For this review, take the finished solid that the model builds, in its own axes (mm). Coordinates: 2 decimals unless noted, no trailing zeros. Write each loop counter-clockwise with the first axis right and the second up, starting at its lowest first coordinate (ties: lowest second). Pieces come first, ordered by that corner, then holes.
```python
from build123d import *

# Parameters (mm, degrees)
PAD_DEPTH     = 3
SKETCH002_R   = 1.95
HOLE_DEPTH    = 3.001
SKETCH_R      = 15
HOLE001_DEPTH = 3.001
SKETCH003_R   = 1.95
HOLE002_DEPTH = 3.001
SKETCH004_R   = 5.7
SKETCH004_R_2 = 4.8
POCKET_DEPTH  = 3.001


with BuildPart() as part:
    # Sketch001 → Pad (new body)
    with BuildSketch(Plane.XY):
        with BuildLine():
            Line((11.5, 190), (11.5, 20))
            ThreePointArc((11.5, 20), (12.525126, 17.525126), (15, 16.5))
            Line((15, 16.5), (120, 16.5))
            ThreePointArc((120, 16.5), (122.474874, 17.525126), (123.5, 20))
            Line((123.5, 20), (123.5, 190))
            ThreePointArc((123.5, 190), (122.474874, 192.474874), (120, 193.5))
            Line((120, 193.5), (15, 193.5))
            ThreePointArc((15, 193.5), (12.525126, 192.474874), (11.5, 190))
        make_face()
    extrude(amount=PAD_DEPTH)

    # Sketch002 → Hole (cut, through all)
    with BuildSketch(Plane.XY):
        with Locations((50, 87.5)):
            Circle(SKETCH002_R)
        with Locations((85, 87.5)):
            Circle(SKETCH002_R)
        with Locations((85, 122.5)):
            Circle(SKETCH002_R)
        with Locations((50, 122.5)):
            Circle(SKETCH002_R)
    extrude(amount=HOLE_DEPTH, mode=Mode.SUBTRACT)

    # Sketch → Hole001 (cut, through all)
    with BuildSketch(Plane.XY):
        with Locations((67.5, 105)):
            Circle(SKETCH_R)
    extrude(amount=HOLE001_DEPTH, mode=Mode.SUBTRACT)

    # Sketch003 → Hole002 (cut, through all)
    with BuildSketch(Plane.XY):
        with Locations((90, 83)):
            Circle(SKETCH003_R)
        with Locations((45, 83)):
            Circle(SKETCH003_R)
        with Locations((45, 128)):
            Circle(SKETCH003_R)
        with Locations((90, 128)):
            Circle(SKETCH003_R)
    extrude(amount=HOLE002_DEPTH, mode=Mode.SUBTRACT)

    # Sketch004 → Pocket (cut, through all)
    with BuildSketch(Plane.XY):
        with Locations((45, 35)):
            Circle(SKETCH004_R)
        with Locations((65, 35)):
            Circle(SKETCH004_R_2)
    extrude(amount=POCKET_DEPTH, mode=Mode.SUBTRACT)


solid = part.part
```
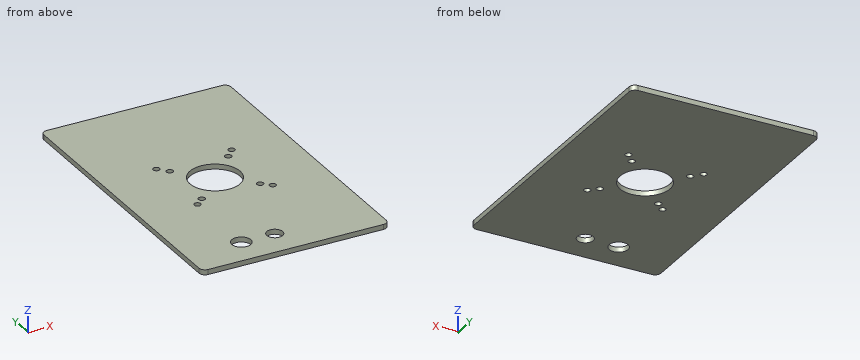
Q1. For probe 1 along Y at (x, z) = (45, 1.6); probe 2 along Y at (x, z) = (85, 1.2); probe 3 along Y at (x, z) = (90, 1.7), list the stretches that pass through material, from the lowest coordinate up.
Ans:
probe 1: y = 16.5 to 29.3, 40.7 to 81.05, 84.95 to 126.05, 129.95 to 193.5
probe 2: y = 16.5 to 85.55, 89.45 to 120.55, 124.45 to 193.5
probe 3: y = 16.5 to 81.05, 84.95 to 126.05, 129.95 to 193.5
Q2. Add section C-C (y = 83). State the section outline as (x, z) points.
Ans:
outline: (11.5, 0) - (43.05, 0) - (43.05, 3) - (11.5, 3) - close; (46.95, 0) - (88.05, 0) - (88.05, 3) - (46.95, 3) - close; (91.95, 0) - (123.5, 0) - (123.5, 3) - (91.95, 3) - close
Q3. Add section A-A (x = 45). State the section outline as (y, z) points, then the cut area to 3 significant figures.
Ans:
outline: (16.5, 0) - (29.3, 0) - (29.3, 3) - (16.5, 3) - close; (40.7, 0) - (81.05, 0) - (81.05, 3) - (40.7, 3) - close; (84.95, 0) - (126.05, 0) - (126.05, 3) - (84.95, 3) - close; (129.95, 0) - (193.5, 0) - (193.5, 3) - (129.95, 3) - close
area: 473 mm2
Q4. Add section B-B (y = 105). State the section outline as (x, z) points.
Ans:
outline: (11.5, 0) - (52.5, 0) - (52.5, 3) - (11.5, 3) - close; (82.5, 0) - (123.5, 0) - (123.5, 3) - (82.5, 3) - close
Q5. Clearance check with a flat-ended pin moving along its axis: pin 1 Ø5 at (x, y) = (85, 122.5) entering from +Z. State where the tip first meets the part, or that it passes through.
Ans:
pin 1: stops at z = 3
Q6. Add section D-D (x = 85). State the section outline as (y, z) points, then the cut area to 3 significant figures.
Ans:
outline: (16.5, 0) - (85.55, 0) - (85.55, 3) - (16.5, 3) - close; (89.45, 0) - (120.55, 0) - (120.55, 3) - (89.45, 3) - close; (124.45, 0) - (193.5, 0) - (193.5, 3) - (124.45, 3) - close
area: 508 mm2
